Check sheet for the modelled part. Datum: model origin and axes. Units: mm. A direction names the side the tool comes from. Give positions to 0.01 mm unless a question says otherwise; leave off trailing zeros. Write each loop counter-clockwise with the first axis right and the second up, starting at its lowest first coordinate (ties: lowest second). Pieces come first, ordered by that corner, then holes. Notation, with made-up numbers: (71, 36.25) -> (81, 36.25) arc R31 ccw to (81, 71.25) -> close; hole circle Ø7 at (73.25, -24.5). An arc over 180 degrees is marked (long way). Answer as a JSON object with one key per item and string values.
from build123d import *

# Parameters (mm, degrees)
SKETCH1_R           = 10
BOSS_EXTRUDE1_DEPTH = 68
SKETCH3_W           = 45
SKETCH3_H           = 38
CUT_EXTRUDE1_DEPTH  = 126
SKETCH4_W           = 75
SKETCH4_H           = 45
SKETCH4_W_2         = 25
CUT_EXTRUDE2_DEPTH  = 53
SKETCH4_2_W         = 25
SKETCH4_2_H         = 45
CUT_EXTRUDE3_DEPTH  = 69
SKETCH5_R           = 6.5
SKETCH5_W           = 25
SKETCH5_H           = 38
CUT_EXTRUDE4_DEPTH  = 16


with BuildPart() as part:
    # Sketch1 → Boss-Extrude1 (new body)
    with BuildSketch(Plane(origin=(0, 0, 0), x_dir=(1, 0, 0), z_dir=(0, 1, 0))):
        Polygon((-50, -30), (50, -30), (75, -30), (75, 30), (50, 30), (-50, 30), align=None)
        Circle(SKETCH1_R, mode=Mode.SUBTRACT)
    extrude(amount=BOSS_EXTRUDE1_DEPTH)

    # Sketch3 → Cut-Extrude1 (cut, through all)
    with BuildSketch(Plane(origin=(75, 0, 0), x_dir=(0, 0, -1), z_dir=(1, 0, 0))):
        with Locations((7.5, 34)):
            Rectangle(SKETCH3_W, SKETCH3_H)
    extrude(amount=-CUT_EXTRUDE1_DEPTH, mode=Mode.SUBTRACT)

    # Sketch4 → Cut-Extrude2 (cut)
    with BuildSketch(Plane(origin=(0, 68, 0), x_dir=(1, 0, 0), z_dir=(0, 1, 0))):
        with Locations((-12.5, -7.5)):
            Rectangle(SKETCH4_W, SKETCH4_H)
        with Locations((62.5, 7.5)):
            Rectangle(SKETCH4_W_2, SKETCH4_H)
    extrude(amount=-CUT_EXTRUDE2_DEPTH, mode=Mode.SUBTRACT)

    # Sketch4<2> → Cut-Extrude3 (cut, through all)
    with BuildSketch(Plane(origin=(0, 68, 0), x_dir=(1, 0, 0), z_dir=(0, 1, 0))):
        with Locations((62.5, 7.5)):
            Rectangle(SKETCH4_2_W, SKETCH4_2_H)
    extrude(amount=-CUT_EXTRUDE3_DEPTH, mode=Mode.SUBTRACT)

    # Sketch5 → Cut-Extrude4 (cut, through all)
    with BuildSketch(Plane(origin=(0, 0, 15), x_dir=(-1, 0, 0), z_dir=(0, 0, -1))):
        with Locations((-63, 15)):
            Circle(SKETCH5_R)
        with Locations((-62.5, 49)):
            Rectangle(SKETCH5_W, SKETCH5_H)
    extrude(amount=-CUT_EXTRUDE4_DEPTH, mode=Mode.SUBTRACT)


solid = part.part
1. Sectioned sample at B-B, the plane z = 0. Enter the section's corners in (x, y), plus the area to 4 significant figures.
Determined:
{"outline": "(-50, 0) -> (-10, 0) -> (-10, 15) -> (-50, 15) -> close; (10, 0) -> (50, 0) -> (50, 15) -> (10, 15) -> close; (25, 53) -> (50, 53) -> (50, 68) -> (25, 68) -> close", "area": "1,575 mm^2"}
2. Sectioned sample at C-C, the plane x = 18. Enter the section's corners in (y, z), plus the area to 4 significant figures.
Determined:
{"outline": "(0, -30) -> (15, -30) -> (15, 30) -> (0, 30) -> close; (53, -30) -> (68, -30) -> (68, -15) -> (53, -15) -> close", "area": "1,125 mm^2"}
3. Access from +Z, -Z, +X, -X, +Y, -Y to the whole of each face (thin tool, end or side, straight path). Record for faces 1 (the face through (-12, 15, 0)), 2 (the face through (-13, 61, -15)), 3 (the face through (12, 53, -17)), 4 (the face through (50, 8, -7)).
Determined:
{"face 1": "-Z, -X", "face 2": "+Z, -X, +Y", "face 3": "-Z, +X, -X", "face 4": "-Z, +X, +Y, -Y"}
4. Go/stop test with flat-tipped pins: P1, Ø10, axis at y = 48.5, z = -9, coming from the +X side; P2, Ø4, axis at x = 1.5, z = 20, coming from the -Y side; P3, Ø18, axis at x = 0, z = 0, coming from the +Y side; P4, Ø7.5, axis at x = 67, z = 21.5, coming from the +Y side. Record where each tip stops, or that it passes through.
Determined:
{"P1": "x = 50", "P2": "y = 0", "P3": "through", "P4": "y = 30"}
5. Sectioned sample at A-A, the plane x = 0. Enter the section's corners in (y, z), plus the area to 3 significant figures.
Determined:
{"outline": "(0, -30) -> (15, -30) -> (15, -10) -> (0, -10) -> close; (0, 10) -> (15, 10) -> (15, 30) -> (0, 30) -> close; (53, -30) -> (68, -30) -> (68, -15) -> (53, -15) -> close", "area": "825 mm^2"}
6. Sectioned sample at D-D, the plane z = 20. Enter the section's corners in (x, y), plus the area to 3 significant figures.
Determined:
{"outline": "(-50, 0) -> (75, 0) -> (75, 30) -> (50, 30) -> (50, 68) -> (25, 68) -> (25, 15) -> (-50, 15) -> close; hole circle Ø13 at (63, 15)", "area": "3,440 mm^2"}
7. Mould release check, pull along X, two halves, no side actions. Record for faces 5 (the face through (56.8, 16.95, 22.4)), 6 (the face through (1, 7, -30)), 7 (the face through (-50, 60, -23)): released by +X, released by -X, zero draft, split by the parting line, or undercut.
Determined:
{"face 5": "undercut", "face 6": "zero draft", "face 7": "released by -X"}
8. Scan lines: L1, parallel to Y at x = 63, z = 20.25; L2, parallel to Z at x = 0, y = 5.5; L3, parallel to Y at x = 33, z = -15.5. Record each from-to range of solid material in increasing order. Write a range as [from, to].
Determined:
{"L1": "[0, 8.5], [21.5, 30]", "L2": "[-30, -10], [10, 30]", "L3": "[0, 15], [53, 68]"}
